```python
from build123d import *

# Parameters (mm, degrees)
SKETCH1_W                      = 50
SKETCH1_H                      = 25
SKETCH1_W_2                    = 40
SKETCH1_H_2                    = 10
BOSS_EXTRUDE1_DEPTH            = 25.2
HOLE1_D                        = 10.2
HOLE1_DEPTH                    = 10
HOLE1_CBORE_D                  = 11.4
HOLE1_CBORE_DEPTH              = 0.6
SKETCH10_W                     = 12.7
SKETCH10_H                     = 25.2
BOSS_EXTRUDE2_DEPTH            = 6
M4_CLEARANCE_HOLE1_D           = 4.5
M4_CLEARANCE_HOLE1_DEPTH       = 11
M4_CLEARANCE_HOLE1_CSINK_D     = 4.55
M4_CLEARANCE_HOLE1_CSINK_ANGLE = 90
SKETCH11_W                     = 20
SKETCH11_H                     = 3.85
CUT_EXTRUDE1_DEPTH             = 42.860363114
FILLET1_R                      = 5


with BuildPart() as part:
    # Sketch1 → Boss-Extrude1 (new body)
    with BuildSketch(Plane(origin=(0, 0, 0), x_dir=(1, 0, 0), z_dir=(0, 1, 0))):
        Rectangle(SKETCH1_W, SKETCH1_H)
        with Locations((0, -2.5)):
            Rectangle(SKETCH1_W_2, SKETCH1_H_2, mode=Mode.SUBTRACT)
    extrude(amount=BOSS_EXTRUDE1_DEPTH)

    # Hole1
    with Locations(Plane.XY.offset(-2.5)):
        with Locations((-11.4, 12.6)):
            CounterBoreHole(HOLE1_D / 2, HOLE1_CBORE_D / 2, HOLE1_CBORE_DEPTH, depth=HOLE1_DEPTH)

    # Sketch10 → Boss-Extrude2 (add)
    with BuildSketch(Plane(origin=(25, 0, 0), x_dir=(0, 0, -1), z_dir=(1, 0, 0))):
        with Locations((0, 12.6)):
            Rectangle(SKETCH10_W, SKETCH10_H)
    extrude(amount=BOSS_EXTRUDE2_DEPTH)

    # M4 Clearance Hole1
    with Locations(Plane.ZY.offset(-20)):
        with Locations((0, 20.1), (0, 5.1)):
            CounterSinkHole(M4_CLEARANCE_HOLE1_D / 2, M4_CLEARANCE_HOLE1_CSINK_D / 2, depth=M4_CLEARANCE_HOLE1_DEPTH, counter_sink_angle=M4_CLEARANCE_HOLE1_CSINK_ANGLE)

    # Sketch11 → Cut-Extrude1 (cut, through all)
    with BuildSketch(Plane(origin=(0, 25.2, 0), x_dir=(1, 0, 0), z_dir=(0, 1, 0))):
        with Locations((10, 4.425)):
            Rectangle(SKETCH11_W, SKETCH11_H)
    extrude(amount=-CUT_EXTRUDE1_DEPTH, mode=Mode.SUBTRACT)

    # Fillet1
    # the kernel refuses this fillet: 5 mm, written as the material it adds along each edge
    with BuildSketch(Plane(origin=(0, 25.2, -6.35), x_dir=(1, 0, 0), z_dir=(0, -1, 0))) as fillet1_piece_1:
        with BuildLine():
            CenterArc((4.865953144, 5), FILLET1_R, 193.297071747, 76.702928253)
            Line((0, 3.85), (0, 0))
            Line((0, 0), (4.865953144, 0))
        make_face()
    extrude(amount=25.2)
    # the kernel refuses this fillet: 5 mm, written as the material it takes off along each edge
    with BuildSketch(Plane(origin=(25, 0, -25), x_dir=(-1, 0, 0), z_dir=(0, 0, 1)), Plane(origin=(25, 0, 6.35), x_dir=(-1, 0, 0), z_dir=(0, 0, 1))) as fillet1_2_piece_1:
        with BuildLine():
            CenterArc((FILLET1_R, -FILLET1_R), FILLET1_R, 90, 90)
            Line((0, -FILLET1_R), (0, 0))
            Line((0, 0), (FILLET1_R, 0))
        make_face()
    extrude(amount=18.65, mode=Mode.SUBTRACT)
    with BuildSketch(Plane(origin=(25, 25.2, -25), x_dir=(-1, 0, 0), z_dir=(0, 0, 1)), Plane(origin=(25, 25.2, 6.35), x_dir=(-1, 0, 0), z_dir=(0, 0, 1))) as fillet1_2_piece_2:
        with BuildLine():
            CenterArc((FILLET1_R, FILLET1_R), FILLET1_R, 180, 90)
            Line((0, FILLET1_R), (0, 0))
            Line((0, 0), (FILLET1_R, 0))
        make_face()
    extrude(amount=18.65, mode=Mode.SUBTRACT)
    with BuildSketch(Plane(origin=(-25, 0, 25), x_dir=(0, 1, 0), z_dir=(0, 0, -1))) as fillet1_2_piece_3:
        with BuildLine():
            CenterArc((FILLET1_R, FILLET1_R), FILLET1_R, 180, 90)
            Line((0, FILLET1_R), (0, 0))
            Line((0, 0), (FILLET1_R, 0))
        make_face()
    extrude(amount=50, mode=Mode.SUBTRACT)
    with BuildSketch(Plane(origin=(-25, 25.2, 25), x_dir=(0, -1, 0), z_dir=(0, 0, -1))) as fillet1_2_piece_4:
        with BuildLine():
            CenterArc((FILLET1_R, -FILLET1_R), FILLET1_R, 90, 90)
            Line((0, -FILLET1_R), (0, 0))
            Line((0, 0), (FILLET1_R, 0))
        make_face()
    extrude(amount=50, mode=Mode.SUBTRACT)


solid = part.part
```
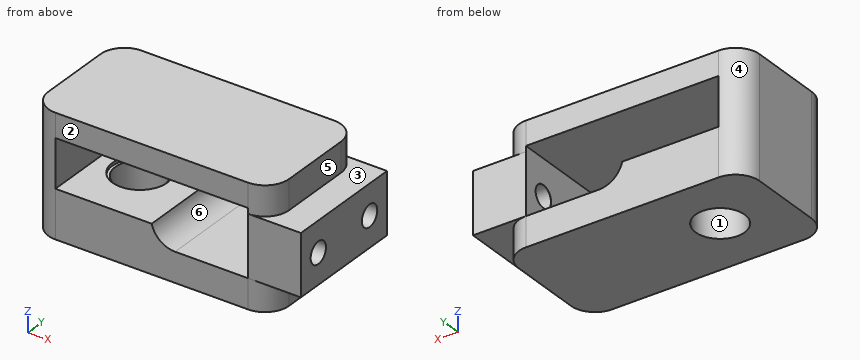
Work out the finished part from the listing and answer in its coordinate system (mm). Face numbers are marked on the shaded views. A direction names the side the tool comes from. Round coordinates to 2 decimals unless told otherwise and drop trailing zeros. Write each loop counter-clockwise with the first axis right and the second up, starting at its lowest first coordinate (ties: lowest second). Pieces come first, ordered by that corner, then holes.
1) Consider probe 1 along Z at (x, y) = (7, 3.5); probe 2 along Y at (x, z) = (28.5, 0); probe 3 along Z at (x, y) = (-2.5, 11). Determine where each line is inside the solid, lowest interval first.
2) A cutting plane is placed at C-C on x = -14.5. Determine the outline of the cut face in (y, z), and give its area (3 significant figures).
3) Determine the mould class of the marked faces 1, 2 and 3 for opening direction Y: pulls with the +Y half, pulls with the -Y half, needs draft (parallel to the pull), parting line crosses it, or undercut.
4) Which of the six approach directions +Z, -Z, +X, -X, +Y, -Y give full straight-line access (tool end or side, diameter ignored) to the marked faces 4, 5 and 6?
5) A cutting plane is placed at A-A on z = 4.25. Determine the outline of the cut face in (x, y), and give its area (3 significant figures).
6) Flat-ended cylindrical pins translate along their axes: P1, Ø1, axis at y = 9.5, z = 7, coming from the +X side; P2, Ø9, axis at x = -11.4, y = 12.6, coming from the -Z side. Find the tip coordinate at first contact, or state that the pin passes through.
7) A cutting plane is placed at B-B on z = 0. Determine the outline of the cut face in (x, y) (3 decimals).
8) A cutting plane is placed at D-D on y = 12.6. Determine the outline of the cut face in (x, z), and give its area (3 significant figures).
Entries:
1. probe 1: z = -12.5 to -6.35, 7.5 to 12.5
1. probe 2: y = 0 to 2.85, 7.35 to 17.85, 22.35 to 25.2
1. probe 3: z = -12.5 to -2.5, 7.5 to 12.5
2. outline: (0, -12.5) - (8.55, -12.5) - (8.55, -3.1) - (7.82, -3.1) - (7.82, -2.5) - (0, -2.5) - close; (0, 7.5) - (25.2, 7.5) - (25.2, 12.5) - (0, 12.5) - close; (16.65, -12.5) - (25.2, -12.5) - (25.2, -2.5) - (17.38, -2.5) - (17.38, -3.1) - (16.65, -3.1) - close
2. area: 296 mm2
3. face 1: undercut
3. face 2: pulls with the -Y half
3. face 3: needs draft
4. face 4: +Z, -Z, -X, +Y
4. face 5: +Z, +X, +Y, -Y
4. face 6: +Y, -Y
5. outline: (-25, 5) arc R5 ccw to (-20, 0) - (-20, 25.2) arc R5 ccw to (-25, 20.2) - close; (20, 0) - (31, 0) - (31, 25.2) - (20, 25.2) - close
5. area: 392 mm2
6. P1: stops at x = 25
6. P2: stops at z = 7.5
7. outline: (-25, 5) arc R5 ccw to (-20, 0) - (-20, 25.2) arc R5 ccw to (-25, 20.2) - close; (20, 0) - (31, 0) - (31, 2.85) - (20.025, 2.85) - (20, 2.825) - close; (20, 7.375) - (20.025, 7.35) - (31, 7.35) - (31, 17.85) - (20.025, 17.85) - (20, 17.825) - close; (20, 22.375) - (20.025, 22.35) - (31, 22.35) - (31, 25.2) - (20, 25.2) - close
8. outline: (-25, -12.5) - (-16.5, -12.5) - (-16.5, -3.1) - (-17.1, -3.1) - (-17.1, -2.5) - (-20, -2.5) - (-20, 7.5) - (20, 7.5) - (20, -6.35) - (4.87, -6.35) arc R5 cw to (0, -2.5) - (-5.7, -2.5) - (-5.7, -3.1) - (-6.3, -3.1) - (-6.3, -12.5) - (25, -12.5) - (25, -6.35) - (31, -6.35) - (31, 6.35) - (25, 6.35) - (25, 12.5) - (-25, 12.5) - close
8. area: 751 mm2
